Answer from the drawing. Dimensions are ordinates in mm from the lowest x, y and z of the part. A direction names the side the tool comes from. Round coordinates to 2 decimals unless told otherwise and drop trailing zeros. Write each loop counter-clockwise with the first axis right and the second up, starting at its lowest first coordinate (ties: lowest second). Pieces come first, ordered by that corner, then holes. Notation, with made-up numbers: (50, 26) - (100, 26) arc R19 cw to (100, 63) - close; hole circle Ø6 at (60, 41). An arc over 180 degrees is marked (long way). One line per item, written item: value. Start each with the question number.
(1) The mould has two halves that part along Y. Classify the marked faces 1, 2, 3 and 4: +Y half, -Y half, draft (parallel to the pull), parting line (faces both ways), or undercut.
(2) Find the intervals of material crossed by L1, parallel to Y at x = 12, z = 11; L2, parallel to X at y = 30, z = 2; L3, parallel to Z at x = 31, y = 28, in increasing order.
(3) For the marked faces 5 and 6, determine the directions among +Z, -Z, +X, -X, +Y, -Y from which every point of the face is accessible in a straight line to the end or side of a thin tool.
(4) A flat-ended cylindrical pin translates along its axis: pin 1 Ø1.5 at (x, y) = (26, 24) entering from -Z. Find the tip coordinate at first contact, or state that the pin passes through.
(5) A cutting plane is placed at A-A, the plane z = 10. Determine the outline of the cut face in (x, y), plus the area to 4 significant figures.
(6) A cutting plane is placed at C-C, the plane y = 25. Determine the outline of the cut face in (x, z), plus the area to 3 significant figures.
(7) A cutting plane is placed at B-B, the plane x = 25. Determine the outline of the cut face in (y, z), plus the area to 3 significant figures.
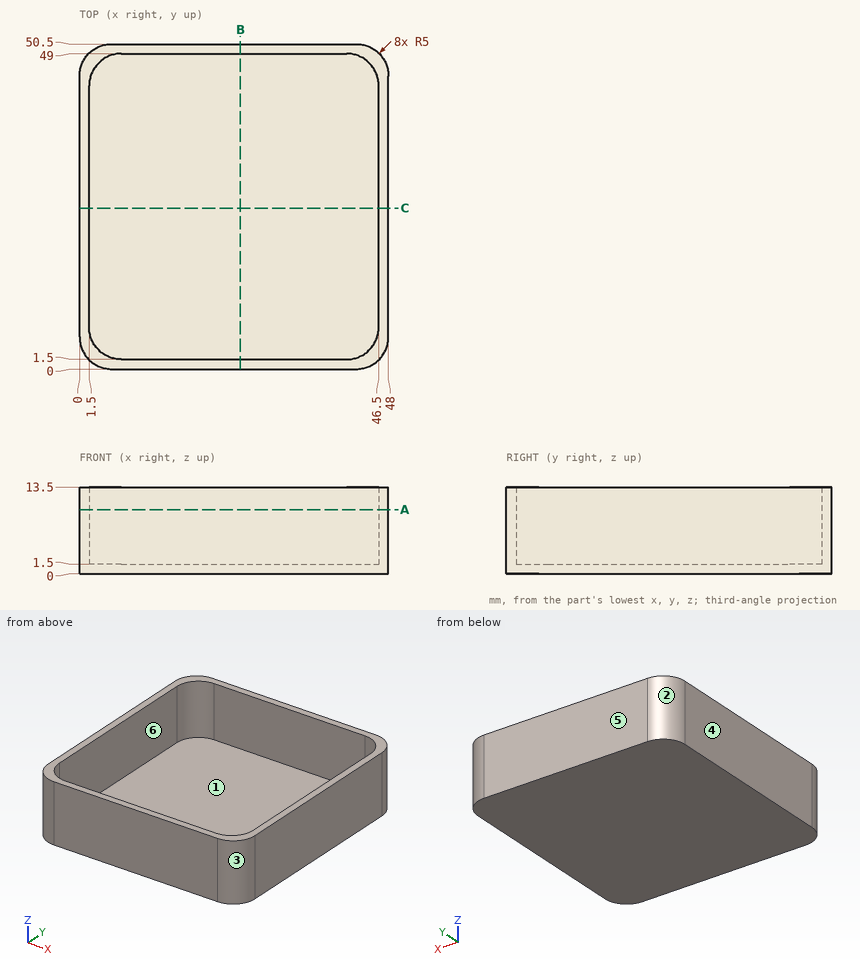
Here are the results:
1. face 1: undercut
1. face 2: +Y half
1. face 3: -Y half
1. face 4: draft
2. L1: 0 to 1.5, 49 to 50.5
2. L2: 0 to 1.5, 46.5 to 48
2. L3: 0 to 1.5
3. face 5: +Z, -Z, +X, -X, +Y
3. face 6: +Z
4. pin 1: z = 0
5. outline: (0, 5) arc R5 ccw to (5, 0) - (43, 0) arc R5 ccw to (48, 5) - (48, 45.5) arc R5 ccw to (43, 50.5) - (5, 50.5) arc R5 ccw to (0, 45.5) - close; hole (1.5, 6.5) arc R5 ccw to (6.5, 1.5) - (41.5, 1.5) arc R5 ccw to (46.5, 6.5) - (46.5, 44) arc R5 ccw to (41.5, 49) - (6.5, 49) arc R5 ccw to (1.5, 44) - close
5. area: 286.5 mm²
6. outline: (0, 0) - (48, 0) - (48, 13.5) - (46.5, 13.5) - (46.5, 1.5) - (1.5, 1.5) - (1.5, 13.5) - (0, 13.5) - close
6. area: 108 mm²
7. outline: (0, 0) - (50.5, 0) - (50.5, 13.5) - (49, 13.5) - (49, 1.5) - (1.5, 1.5) - (1.5, 13.5) - (0, 13.5) - close
7. area: 112 mm²
